The figure shows three views and two pictorial views of one solid part (mm, origin at its lowest corner). Answer the questions. A direction names the side the tool comes from. Coordinates: 2 decimals unless noted, no trailing zeros. Write each loop counter-clockwise with the first axis right and the second up, starting at its lowest first coordinate (ties: lowest second). Pieces come first, ordered by that corner, then holes. Notation, with made-up numbers: M 28.5,56.25 L 87.5,56.25 A18 ccw 87.5,61.25 Z; hole C 82,50 d1. An arc over 180 degrees is marked long. Write item = value, one per line.
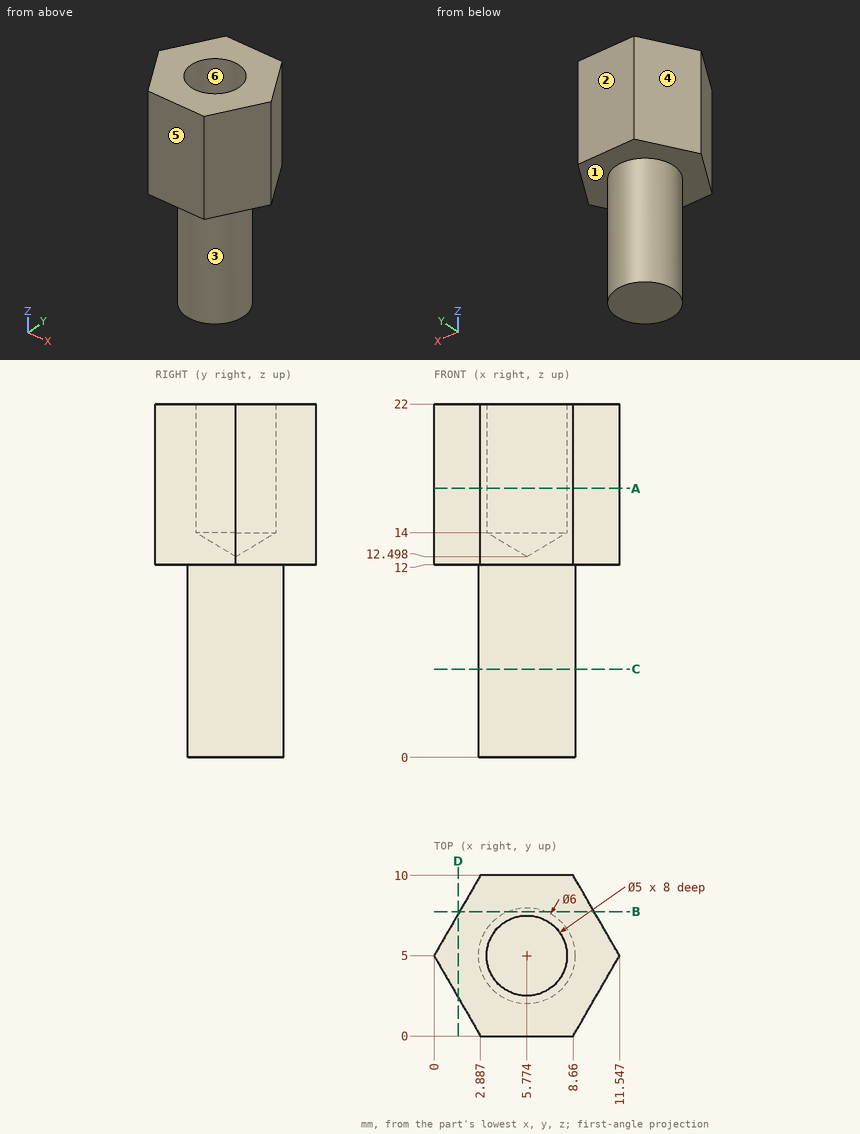
Item 1: Find section C-C (z = 5.5). Determine the outline of the cut face in (x, y), and give its area (3 significant figures).
Worked answers:
outline = C 5.77,5 d6
area = 28.3 mm²
Item 2: Find section D-D (x = 1.5). Determine the outline of the cut face in (y, z).
Worked answers:
outline = M 2.4,12 L 7.6,12 L 7.6,22 L 2.4,22 Z
Item 3: For a pull along Y with two mould halves and no side action, classify the marked faces 3, 4, 5 and 6 as released by +Y, released by -Y, zero draft, split by the parting line, or undercut.
Worked answers:
face_3 = split by the parting line
face_4 = released by +Y
face_5 = released by -Y
face_6 = undercut
Item 4: Which of the six approach directions +Z, -Z, +X, -X, +Y, -Y give full straight-line access (tool end or side, diameter ignored) to the marked faces 1 and 2?
Worked answers:
face_1 = -Z
face_2 = +Z, -Z, +X, -X, +Y
Item 5: Consider line 1 along Z through (x, y) = (5.25, 1.5); line 2 along X through (y, z) = (3.75, 21) (1 decimal); line 3 along Y through (x, z) = (8, 16.5) (1 decimal). Determine where each line is inside the solid, lowest interval first. Write a range as from..to.
Worked answers:
line_1 = 12..22
line_2 = 0.7..3.6, 7.9..10.8
line_3 = 0..3.9, 6.1..10
Item 6: Flat-ended cylindrical pins translate along their axes: pin 1 (1.5 mm diameter, centred on y = 4, z = 9.5, fed in from -X); pin 2 (6 mm diameter, centred on x = 4.5, z = 11, fed in from +Y); pin 3 (1 mm diameter, centred on x = 3.5, z = 3, fed in from +Y); pin 4 (6 mm diameter, centred on x = 2.5, z = 4.5, fed in from +Y). Find the tip coordinate at first contact, or state that the pin passes through.
Worked answers:
pin_1 = 2.78
pin_2 = 10
pin_3 = 7.42
pin_4 = 7.99
Item 7: Find section B-B (y = 7.75). Determine the outline of the cut face in (x, z) (1 decimal).
Worked answers:
outline = M 1.6,12 L 4.6,12 L 4.6,0 L 7,0 L 7,12 L 10,12 L 10,22 L 1.6,22 Z
Item 8: Find section A-A (z = 16.75). Determine the outline of the cut face in (x, y).
Worked answers:
outline = M 0,5 L 2.89,0 L 8.66,0 L 11.55,5 L 8.66,10 L 2.89,10 Z; hole C 5.77,5 d5
